Autodesk Inventor part; units mm, degrees
ref_plane "Start plane" through (0, 0, 0) normal (0, 0, 1) x (1, 0, 0)
ref_plane "End plane" through (0, 0, 1022.35) normal (0, 0, 1) x (1, 0, 0)
ref_plane "YZ Plane" through (0, 0, 0) normal (1, 0, 0) x (0, 1, 0)
ref_plane "Start plane" through (0, 0, 0) normal (0, 0, 1) x (1, 0, 0)
ref_plane "End plane" through (0, 0, 1022.35) normal (0, 0, 1) x (1, 0, 0)
sketch "Sketch" plane through (0, 0, 0) normal (0, 0, 1) x (1, 0, 0)
  line L0 (0, 76.2) -> (0, 0)
  line L1 (0, 0) -> (50.8, 0)
  line L2 (50.8, 0) -> (50.8, 2.7625)
  line L3 (48.8, 4.7625) -> (12.6365, 4.7625)
  line L4 (4.7625, 12.6365) -> (4.7625, 74.2)
  line L5 (2.7625, 76.2) -> (0, 76.2)
  line L6 (-7.0414, 0) -> (21.5385, 0) construction
  line L7 (0, -8.0414) -> (0, 34.5385) construction
  arc A0 (4.7625, 12.6365) -> (12.6365, 4.7625) centre (12.6365, 12.6365) ccw
  arc A1 (50.8, 2.7625) -> (48.8, 4.7625) centre (48.8, 2.7625) ccw
  arc A2 (4.7625, 74.2) -> (2.7625, 76.2) centre (2.7625, 74.2) ccw
  line L8 (0, 93.5453) -> (0, -24.9725) construction
  line L9 (-18.6925, 0) -> (62.8653, 0) construction
  point P0 (50.8, 4.7625)
  point P1 (4.7625, 4.7625)
  point P2 (4.7625, 76.2)
  dimension "d12" = 4.7625
  dimension "d13" = 76.2
  dimension "d14" = 50.8
  dimension "d15" = 0
  dimension "d16" = 4.7625
  dimension "d17" = 0
  dimension "d18" = 7.874
  dimension "d19" = 2
extrude "Body" add sketch "Sketch" along normal up to surface (1022.35 mm away) from surface at 0
equation "\"d12\" = G_T"
equation "\"d13\" = G_H"
equation "\"d14\" = G_W"
equation "\"d16\" = G_T"
equation "\"d18\" = G_IR"
equation "\"d4\" = G_L"
equation "\"G_W\" = 50.8"
equation "\"G_H\" = 76.2"
equation "\"G_T\" = 4.7625"
equation "\"G_ER\" = 4.064"
equation "\"G_IR\" = 7.874"
equation "\"G_L\" = B_L + G_OFFSET_START + G_OFFSET_END"
equation "\"ex\" = 0"
equation "\"ey\" = 0"
equation "\"G_OFFSET_START\" = 0"
equation "\"G_OFFSET_END\" = 0"
equation "\"d21\" = G_OFFSET_END + B_L"
equation "\"B_L\" = 1022.35"
properties part number "ANSI L 3 x 2 x 3_16 00000005"
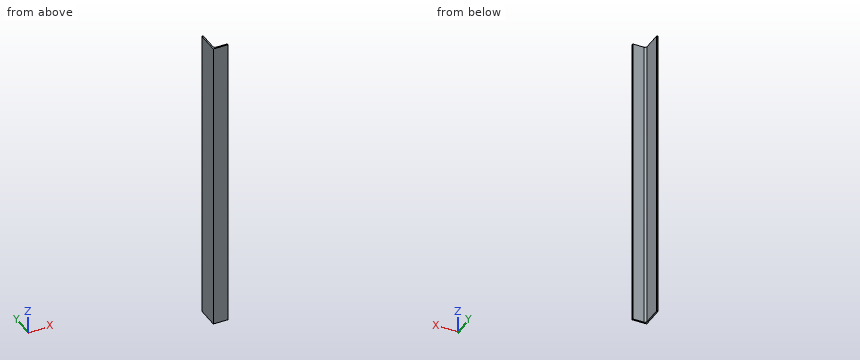
Source: CAD feature listing. Evaluate the final solid. Frame: model axes, mm. Coordinates: 2 decimals unless noted, no trailing zeros. Order: outer loops, then holes, each group sorted by start corner. A loop starts at its lowest first (then second) coordinate and runs counter-clockwise, first axis right, second up. Notation, with made-up numbers: M -34,41 L -16,41 A16 cw -16,48 Z; hole C -14,68 d7. An arc over 180 degrees is marked long. Write each question's results on one line, items separated by ' | '. Start each with the question number.
Item 1: Cut plane B-B (x = 25.5). Return loops of the section in (y, z).
Item 2: Cut plane A-A (z = 388). Return loops of the section in (x, y), and give its area (3 significant figures).
Item 3: First-contact query: pin 1 Ø3 at (y, z) = (48.5, 196) entering from +X; pin 2 Ø3 at (x, z) = (21, 567.5) entering from +Y. Flat tips, straight axial feed; report the tip coordinate or a pass-through.
Item 4: Line query: probe 1 along X at (y, z) = (29, 777.5); probe 2 along Y at (x, z) = (7.5, 481). Output: solid intervals per line, ascending.
Checked values:
1) outline: M 0,0 L 4.76,0 L 4.76,1022.35 L 0,1022.35 Z
2) outline: M 0,0 L 50.8,0 L 50.8,2.76 A2 ccw 48.8,4.76 L 12.64,4.76 A7.87 cw 4.76,12.64 L 4.76,74.2 A2 ccw 2.76,76.2 L 0,76.2 Z | area: 594 mm2
3) pin 1: stops at x = 4.76 | pin 2: stops at y = 4.76
4) probe 1: x = 0 to 4.76 | probe 2: y = 0 to 6.67
